Build history of the part. All positions in model axes, mm. A direction names the side the tool comes from. Give positions to 0.01 mm unless a question says otherwise; leave off trailing zeros. Order: outer loops, then holes, each group sorted by start corner. A loop starts at its lowest first (then second) coordinate and runs counter-clockwise, first axis right, second up. Notation, with made-up numbers: (69.25, 29) - (87.25, 29) arc R36 ccw to (87.25, 63) - close; hole circle Ø1 at (64.5, 84.25). An arc over 180 degrees is marked (long way). Write each question's results on one line, items separated by ' | '. Start each with the question number.
1) Cut at D-D on x = 24.85. State how many separate pieces and enclosed holes the cut face has, plus the area to 3 significant figures.
2) Cut at A-A on y = 10. List the corners of the cut face in (x, z).
3) Drop flat-ended pins along their axis: pin 1 Ø4.5 at (x, y) = (24.85, -10) entering from -Z; pin 2 Ø1.5 at (x, y) = (17, 33.5) entering from +Z; pin 3 Ø11 at (x, z) = (38.5, -13) entering from +Y; pin 4 Ø6.5 at (x, z) = (14, -8) entering from -Y. Give the stop position or say it passes through.
4) Tool access for faces 1 (the face through (21, 12, 0)), 2 (the face through (15, -30, 0)), 3 (the face through (26.519, -9.474, 1.479)): list every direction of +Z, -Z, +X, -X, +Y, -Y with a clear straight run to the whole face (end or side of a thin tool).
5) Cut at C-C on z = -18.25. List the corners of the cut face in (x, y), plus the area to 3 significant figures.
6) Two-plate mould, pull along Y, no slides. Class faces 4 (the face through (21, 1, 3)), 5 (the face through (5, 50.632, 1)), 6 (the face through (9.622, -8.265, 1.479)), 7 (the face through (28, -16.873, -11)): +Y half, -Y half, draft (parallel to the pull), parting line (faces both ways), or undercut.
7) Cut at B-B on x = 6. List the corners of the cut face in (y, z), plus the area to 3 significant figures.
8) Drill centre lines: line 1 along Y through (x, z) = (24.85, 1.4); line 2 along Z through (x, y) = (8, 21); line 3 along Y through (x, z) = (22, -10.25). Where is each one in solid material? Low to high. Write a range as from..to.
from build123d import *

# Parameters (mm, degrees)
SKETCH3_R           = 1.75
BOSS_EXTRUDE2_DEPTH = 3
SKETCH4_W           = 54.71275589
SKETCH4_H           = 3.111536519
BOSS_EXTRUDE3_DEPTH = 22


with BuildPart() as part:
    # Sketch3 → Boss-Extrude2 (new body)
    with BuildSketch(Plane.XY):
        with BuildLine():
            Line((0.033369184, 50.631957294), (0.033369184, -50.424600046))
            Line((0.033369184, -50.424600046), (9.85, -50.631957294))
            add(Edge.make_bspline(
                [(54.746125074, -16.873198091), (45.78853614, -21.288615011), (21.037768937, -20.539930575), (11.485294324, -41.9878824), (9.85, -50.631957294)],
                knots=[0, 0, 0, 0, 0.5491041, 1, 1, 1, 1], degree=3))
            Line((54.746125074, -16.873198091), (54.746125074, 16.873198091))
            add(Edge.make_bspline(
                [(54.746125074, 16.873198091), (45.78853614, 21.288615011), (21.037768937, 20.539930575), (11.485294324, 41.9878824), (9.85, 50.631957294)],
                knots=[0, 0, 0, 0, 0.5491041, 1, 1, 1, 1], degree=3))
            Line((9.85, 50.631957294), (0.033369184, 50.631957294))
        make_face()
        with Locations((9.85, 10)):
            Circle(SKETCH3_R, mode=Mode.SUBTRACT)
        with Locations((24.85, 10)):
            Circle(SKETCH3_R, mode=Mode.SUBTRACT)
        with Locations((24.85, -10)):
            Circle(SKETCH3_R, mode=Mode.SUBTRACT)
        with Locations((9.85, -10)):
            Circle(SKETCH3_R, mode=Mode.SUBTRACT)
    extrude(amount=BOSS_EXTRUDE2_DEPTH)

    # Sketch4 → Boss-Extrude3 (add)
    with BuildSketch(Plane(origin=(0, 0, 0), x_dir=(-1, 0, 0), z_dir=(0, 0, -1))):
        with Locations((-27.389747129, -15.317429832)):
            Rectangle(SKETCH4_W, SKETCH4_H)
    extrude(amount=BOSS_EXTRUDE3_DEPTH)


solid = part.part
Results:
1) separate pieces: 3 | enclosed holes: 0 | area: 204 mm^2
2) outline: (0.03, 0) - (8.1, 0) - (8.1, 3) - (0.03, 3) - close; (11.6, 0) - (23.1, 0) - (23.1, 3) - (11.6, 3) - close; (26.6, 0) - (54.75, 0) - (54.75, 3) - (26.6, 3) - close
3) pin 1: z = 0 | pin 2: z = 3 | pin 3: y = -13.76 | pin 4: y = -16.87
4) face 1: -Z, +X, -X, +Y | face 2: -Z, +X, -X, -Y | face 3: +Z, -Z
5) outline: (0.03, -16.87) - (54.75, -16.87) - (54.75, -13.76) - (0.03, -13.76) - close | area: 170 mm^2
6) face 4: draft | face 5: +Y half | face 6: undercut | face 7: -Y half
7) outline: (-50.55, 0) - (-16.87, 0) - (-16.87, -22) - (-13.76, -22) - (-13.76, 0) - (50.63, 0) - (50.63, 3) - (-50.55, 3) - close | area: 372 mm^2
8) line 1: -26.1..-11.75, -8.25..8.25, 11.75..26.1 | line 2: 0..3 | line 3: -16.87..-13.76
